Geometry check sheet. Reference: the model listing, model coordinates, mm. Face numbers are marked on the shaded views. A direction names the side the tool comes from. Give positions to 0.01 mm unless a question says otherwise; leave off trailing zeros. Loops run counter-clockwise (first coordinate to the right, second up) from the corner with the lowest first, then second, coordinate; pieces in that order, holes last. Notation, with made-up numbers: (46, 2.25) -> (89, 2.25) arc R28 ccw to (89, 29.25) -> close; hole circle Ø3 at (18.25, -18.75). An arc over 180 degrees is marked (long way). Answer as a JSON object with one key per item and string values.
from build123d import *

# Parameters (mm, degrees)
SKETCH2_W                                      = 95
SKETCH2_H                                      = 46.3
BOSS_EXTRUDE1_DEPTH                            = 7.5
SKETCH3_W                                      = 10
SKETCH3_H                                      = 5
SKETCH3_W_2                                    = 19.5
SKETCH3_H_2                                    = 46.3
BOSS_EXTRUDE2_DEPTH                            = 3
SKETCH4_W                                      = 56
SKETCH4_H                                      = 15
SKETCH4_W_2                                    = 20.5
BOSS_EXTRUDE3_DEPTH                            = 6
CSK_FOR_6_FLAT_HEAD_MACHINE_SCREW1_D           = 3.7973
CSK_FOR_6_FLAT_HEAD_MACHINE_SCREW1_CSINK_D     = 7.0866
CSK_FOR_6_FLAT_HEAD_MACHINE_SCREW1_CSINK_ANGLE = 82
CSK_FOR_6_FLAT_HEAD_MACHINE_SCREW2_D           = 3.7973
CSK_FOR_6_FLAT_HEAD_MACHINE_SCREW2_CSINK_D     = 7.0866
CSK_FOR_6_FLAT_HEAD_MACHINE_SCREW2_CSINK_ANGLE = 82
SKETCH18_W                                     = 15
SKETCH18_H                                     = 25.808879712
CUT_EXTRUDE4_DEPTH                             = 6
SKETCH19_W                                     = 20.5
SKETCH19_H                                     = 6
CUT_EXTRUDE5_DEPTH                             = 16.85
CUT_EXTRUDE5_DEPTH_BACK                        = 0.5


with BuildPart() as part:
    # Sketch2 → Boss-Extrude1 (new body)
    with BuildSketch(Plane.XY):
        Rectangle(SKETCH2_W, SKETCH2_H)
    extrude(amount=-BOSS_EXTRUDE1_DEPTH)

    # Sketch3 → Boss-Extrude2 (add)
    with BuildSketch(Plane.XY):
        Rectangle(SKETCH3_W, SKETCH3_H)
        with Locations((37.75, 0)):
            Rectangle(SKETCH3_W_2, SKETCH3_H_2)
        with Locations((-37.75, 0)):
            Rectangle(SKETCH3_W_2, SKETCH3_H_2)
    extrude(amount=BOSS_EXTRUDE2_DEPTH)

    # Sketch4 → Boss-Extrude3 (add)
    with BuildSketch(Plane.XY):
        with Locations((0, -15.65)):
            Rectangle(SKETCH4_W, SKETCH4_H)
        with Locations((17.75, 15.65)):
            Rectangle(SKETCH4_W_2, SKETCH4_H)
        with Locations((-17.75, 15.65)):
            Rectangle(SKETCH4_W_2, SKETCH4_H)
    extrude(amount=BOSS_EXTRUDE3_DEPTH)

    # CSK for #6 Flat Head Machine Screw1 (through all)
    with Locations(Plane.XY):
        with Locations((16.5, 0), (-16.5, 0)):
            CounterSinkHole(CSK_FOR_6_FLAT_HEAD_MACHINE_SCREW1_D / 2, CSK_FOR_6_FLAT_HEAD_MACHINE_SCREW1_CSINK_D / 2, counter_sink_angle=CSK_FOR_6_FLAT_HEAD_MACHINE_SCREW1_CSINK_ANGLE)

    # CSK for #6 Flat Head Machine Screw2 (through all)
    with Locations(Plane(origin=(0, 0, -7.5), x_dir=(-1, 0, 0), z_dir=(0, 0, -1))):
        with Locations((42.25, 11.575), (42.25, -11.575), (-42.25, 11.575), (-42.25, -11.575)):
            CounterSinkHole(CSK_FOR_6_FLAT_HEAD_MACHINE_SCREW2_D / 2, CSK_FOR_6_FLAT_HEAD_MACHINE_SCREW2_CSINK_D / 2, counter_sink_angle=CSK_FOR_6_FLAT_HEAD_MACHINE_SCREW2_CSINK_ANGLE)

    # Sketch18 → Cut-Extrude4 (cut)
    with BuildSketch(Plane.XY):
        with Locations((0, -19.186864523)):
            Rectangle(SKETCH18_W, SKETCH18_H)
    extrude(amount=CUT_EXTRUDE4_DEPTH, mode=Mode.SUBTRACT)

    # Sketch19 → Cut-Extrude5 (cut, two sides)
    with BuildSketch(Plane.XZ.offset(-8.15)) as cut_extrude5_sk:
        with Locations((-17.75, 3)):
            Rectangle(SKETCH19_W, SKETCH19_H)
        with Locations((17.75, 3)):
            Rectangle(SKETCH19_W, SKETCH19_H)
    extrude(amount=CUT_EXTRUDE5_DEPTH, mode=Mode.SUBTRACT)
    extrude(cut_extrude5_sk.sketch, amount=-CUT_EXTRUDE5_DEPTH_BACK, mode=Mode.SUBTRACT)


solid = part.part
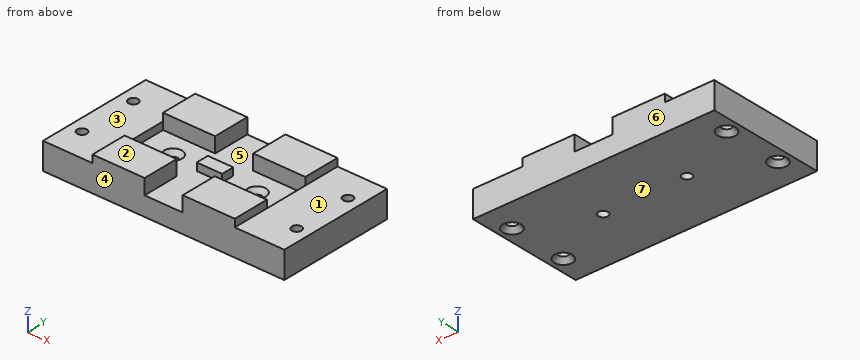
1) Section check B-B on y = 0. Record the cut outline in (x, z).
Geometry check:
{"outline": "(-47.5, -7.5) -> (-18.4, -7.5) -> (-18.4, -1.89) -> (-20.04, 0) -> (-28, 0) -> (-28, 3) -> (-47.5, 3) -> close; (-14.6, -7.5) -> (14.6, -7.5) -> (14.6, -1.89) -> (12.96, 0) -> (5, 0) -> (5, 3) -> (-5, 3) -> (-5, 0) -> (-12.96, 0) -> (-14.6, -1.89) -> close; (18.4, -7.5) -> (47.5, -7.5) -> (47.5, 3) -> (28, 3) -> (28, 0) -> (20.04, 0) -> (18.4, -1.89) -> close"}
2) Section check C-C on x = 26.5. Record the cut outline in (y, z).
Geometry check:
{"outline": "(-23.15, -7.5) -> (23.15, -7.5) -> (23.15, 6) -> (8.65, 6) -> (8.65, 0) -> (-8.7, 0) -> (-8.7, 6) -> (-23.15, 6) -> close"}
3) Section check D-D on y = 20. Record the cut outline in (x, z).
Geometry check:
{"outline": "(-47.5, -7.5) -> (47.5, -7.5) -> (47.5, 3) -> (28, 3) -> (28, 6) -> (7.5, 6) -> (7.5, 0) -> (-7.5, 0) -> (-7.5, 6) -> (-28, 6) -> (-28, 3) -> (-47.5, 3) -> close"}
4) Material ranges on line 1 along X through (y, z) = (0, -5.2); line 2 along Y through (x, z) = (-42.25, 0); line 3 along X through (y, z) = (5.5, 1.5), recorded low to high. Write a range as from..to.
Geometry check:
{"line 1": "x = -47.5..-18.4, -14.6..14.6, 18.4..47.5", "line 2": "y = -23.15..-13.47, -9.68..9.68, 13.47..23.15", "line 3": "x = -47.5..-28, 28..47.5"}
5) Section check A-A on x = -42.25. Record the cut outline in (y, z).
Geometry check:
{"outline": "(-23.15, -7.5) -> (-15.12, -7.5) -> (-13.47, -5.61) -> (-13.47, 3) -> (-23.15, 3) -> close; (-9.68, -5.61) -> (-8.03, -7.5) -> (8.03, -7.5) -> (9.68, -5.61) -> (9.68, 3) -> (-9.68, 3) -> close; (13.47, -5.61) -> (15.12, -7.5) -> (23.15, -7.5) -> (23.15, 3) -> (13.47, 3) -> close"}
6) Tool access check on the marked faces 1, 2 and 3. Record the directions out of +Z, -Z, +X, -X, +Y, -Y that give a thin tool (end or side, any length) a straight path to the whole face; none if there is none.
Geometry check:
{"face 1": "+Z, +X, +Y, -Y", "face 2": "+Z, +X, -X, +Y, -Y", "face 3": "+Z, -X, +Y, -Y"}
7) Draft check along Y on the marked faces 4, 5, 6 and 7. Enter one of: pulls with the +Y half, pulls with the -Y half, needs draft (parallel to the pull), parting line crosses it, or undercut.
Geometry check:
{"face 4": "pulls with the -Y half", "face 5": "undercut", "face 6": "pulls with the +Y half", "face 7": "needs draft"}
8) Depth check by flat-ended pin: P1, Ø2.5, axis at x = 42.25, y = -11.575, coming from the -Z side; P2, Ø15.5, axis at x = -41, y = 2.5, coming from the +Z side; P3, Ø3.5, axis at y = -13.5, z = 4.5, coming from the -X side; P4, Ø4.5, axis at x = 16.5, y = 0, coming from the +Z side. Enter the tip coordinate at first touch or a pass-through.
Geometry check:
{"P1": "passes through", "P2": "stops at z = 3", "P3": "stops at x = -47.5", "P4": "stops at z = -1.49"}
